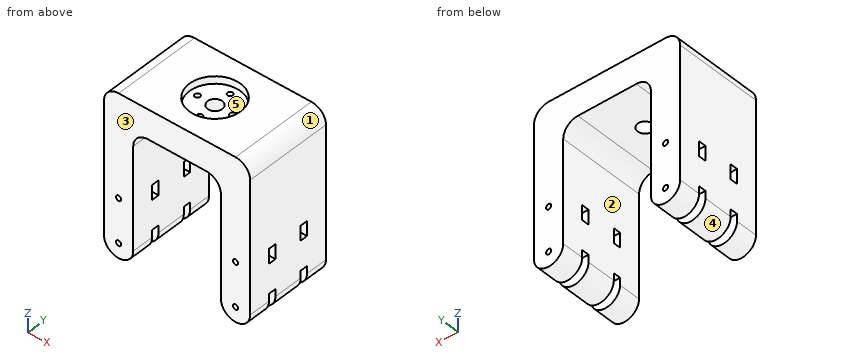
```python
from build123d import *

# Parameters (mm, degrees)
BOSS_EXTRUDE1_DEPTH     = 30
FILLET1_R               = 10
CUT_EXTRUDE1_DEPTH      = 125.49899598
CUT_EXTRUDE1_DEPTH_BACK = 125.49899598
SKETCH3_R               = 5
SKETCH4_R               = 17.5
CUT_EXTRUDE2_DEPTH      = 5
SKETCH5_R               = 1.8
CUT_EXTRUDE3_DEPTH      = 5
CIRPATTERN1_COUNT       = 4
SKETCH6_R               = 1.8
CUT_EXTRUDE4_DEPTH      = 135.907375632
SKETCH7_W               = 20
SKETCH7_H               = 10
CUT_EXTRUDE5_DEPTH      = 5
MIRROR2_COPY_1_SKETCH_W = 20
MIRROR2_COPY_1_SKETCH_H = 10
MIRROR2_COPY_1_DEPTH    = 5


with BuildPart() as part:
    # Sketch1 → Boss-Extrude1 (new, symmetric)
    with BuildSketch(Plane(origin=(0, 0, 0), x_dir=(1, 0, 0), z_dir=(0, 1, 0))):
        with BuildLine():
            Line((-50, 0), (50, 0))
            Line((50, 0), (50, 100))
            ThreePointArc((50, 100), (40, 110), (30, 100))
            Line((30, 100), (30, 20))
            Line((30, 20), (-30, 20))
            Line((-30, 20), (-30, 100))
            ThreePointArc((-30, 100), (-40, 110), (-50, 100))
            Line((-50, 100), (-50, 0))
        make_face()
    extrude(amount=BOSS_EXTRUDE1_DEPTH, both=True)

    # Fillet1
    fillet1_edges = [part.edges().sort_by_distance(p)[0] for p in [
        (50, 0, 0),
        (-50, 0, 0),
        (-30, 0, -20),
        (30, 0, -20),
    ]]
    fillet(fillet1_edges, radius=FILLET1_R)

    # Sketch3 → Cut-Extrude1 (cut, two sides: drawn at the far end of the back side and taken through both)
    with BuildSketch(Plane.XY.offset(-CUT_EXTRUDE1_DEPTH_BACK)):
        Circle(SKETCH3_R)
    extrude(amount=CUT_EXTRUDE1_DEPTH + CUT_EXTRUDE1_DEPTH_BACK, mode=Mode.SUBTRACT)

    # Sketch4 → Cut-Extrude2 (cut)
    with BuildSketch(Plane.XY):
        Circle(SKETCH4_R)
    extrude(amount=-CUT_EXTRUDE2_DEPTH, mode=Mode.SUBTRACT)

    # Sketch5 → Cut-Extrude3 (cut)
    with BuildSketch(Plane.XY.offset(-5)):
        with Locations((0, -12)):
            Circle(SKETCH5_R)
    cut_extrude3 = extrude(amount=-CUT_EXTRUDE3_DEPTH, mode=Mode.SUBTRACT)

    # CirPattern1: Cut-Extrude3 ×4 about axis
    cirpattern1_axis = Axis((0, 0, 0), (0, 0, 1))
    for i in range(1, CIRPATTERN1_COUNT):
        add(cut_extrude3.rotate(cirpattern1_axis, i * 360 / CIRPATTERN1_COUNT), mode=Mode.SUBTRACT)

    # Sketch6 → Cut-Extrude4 (cut, through all)
    with BuildSketch(Plane(origin=(0, 30, 0), x_dir=(1, 0, 0), z_dir=(0, 1, 0))):
        with Locations(Location((-40, 100, 0), (0, 0, 270))):
            Circle(SKETCH6_R)
        with Locations(Location((-40, 70, 0), (0, 0, 270))):
            Circle(SKETCH6_R)
    cut_extrude4 = extrude(amount=-CUT_EXTRUDE4_DEPTH, mode=Mode.SUBTRACT)

    # Sketch7 → Cut-Extrude5 (cut)
    with BuildSketch(Plane(origin=(0, 15, 0), x_dir=(1, 0, 0), z_dir=(0, 1, 0))):
        with BuildLine():
            Line((-50, 105), (-50, 95))
            Line((-50, 95), (-30, 95))
            Line((-30, 95), (-30, 105))
            ThreePointArc((-30, 105), (-40, 115), (-50, 105))
        make_face()
        with Locations((-40, 70)):
            Rectangle(SKETCH7_W, SKETCH7_H)
    cut_extrude5 = extrude(amount=-CUT_EXTRUDE5_DEPTH, mode=Mode.SUBTRACT)

    # Mirror1: Cut-Extrude5 across plane
    add(cut_extrude5.mirror(Plane.ZX), mode=Mode.SUBTRACT)

    # Mirror2: Cut-Extrude4, Cut-Extrude5 across plane
    add(cut_extrude4.mirror(Plane(origin=(0, 0, 0), x_dir=(0, 0, 1), z_dir=(1, 0, 0))), mode=Mode.SUBTRACT)
    add(cut_extrude5.mirror(Plane(origin=(0, 0, 0), x_dir=(0, 0, 1), z_dir=(1, 0, 0))), mode=Mode.SUBTRACT)

    # Mirror2 copy 1 sketch → Mirror2 copy 1 (cut)
    with BuildSketch(Plane(origin=(0, -15, 0), x_dir=(-1, 0, 0), z_dir=(0, -1, 0))):
        with BuildLine():
            Line((-50, 105), (-50, 95))
            Line((-50, 95), (-30, 95))
            Line((-30, 95), (-30, 105))
            ThreePointArc((-30, 105), (-40, 115), (-50, 105))
        make_face()
        with Locations((-40, 70)):
            Rectangle(MIRROR2_COPY_1_SKETCH_W, MIRROR2_COPY_1_SKETCH_H)
    extrude(amount=-MIRROR2_COPY_1_DEPTH, mode=Mode.SUBTRACT)


solid = part.part
```
Work out the finished part from the listing and answer in its coordinate system (mm). Face numbers are marked on the shaded views. A direction names the side the tool comes from. Round coordinates to 2 decimals unless told otherwise and drop trailing zeros. Order: outer loops, then holes, each group sorted by start corner. A loop starts at its lowest first (then second) coordinate and runs counter-clockwise, first axis right, second up.
Q1. A tool of negligible diameter and unlimited length cuts with its end or side. For the marked faces 1 and 2, from which of +Z, -Z, +X, -X, +Y, -Y can it reach the whole face along a straight path? Write none if from no direction.
Solution:
face 1: +Z, +X, +Y, -Y
face 2: -Z, +Y, -Y
Q2. The mould has two halves that part along Y. Classify the marked faces 3, 4 and 5: pulls with the +Y half, pulls with the -Y half, needs draft (parallel to the pull), parting line crosses it, or undercut.
Solution:
face 3: pulls with the -Y half
face 4: needs draft
face 5: undercut
Q3. Given pin 1 Ø1.8 at (x, y) = (0.5, 11.5) entering from +Z; pin 2 Ø3 at (x, z) = (-40, -100) entering from -Y; pin 3 Ø1.5 at (x, y) = (-42, 12.5) entering from -Z; pin 4 Ø4 at (x, y) = (-44, 11.5) entering from -Z (3 decimals), each flat-ended and moving along its own axis, determine where each tip first touches the part or whether it passes through.
Solution:
pin 1: stops at z = -10
pin 2: passes through
pin 3: stops at z = -95
pin 4: stops at z = -109.635
Q4. A cutting plane is placed at C-C, the plane z = -53.5. Determine the outline of the cut face in (x, y).
Solution:
outline: (-50, -30) - (-30, -30) - (-30, 30) - (-50, 30) - close; (30, -30) - (50, -30) - (50, 30) - (30, 30) - close
Q5. Find the intervals of material crossed by line 1 along X through (y, z) = (24.75, -70); line 2 along Y through (x, z) = (0, -7); line 3 along Y through (x, z) = (30.5, -100), in increasing order.
Solution:
line 1: x = -50 to -41.8, -38.2 to -30, 30 to 38.2, 41.8 to 50
line 2: y = -30 to -13.8, -10.2 to -5, 5 to 10.2, 13.8 to 30
line 3: y = -30 to -15, -10 to 10, 15 to 30
Q6. A cutting plane is placed at B-B, the plane x = 0. Determine the outline of the cut face in (y, z), then the cut area to 3 significant figures.
Solution:
outline: (-30, -20) - (-5, -20) - (-5, -5) - (-10.2, -5) - (-10.2, -10) - (-13.8, -10) - (-13.8, -5) - (-17.5, -5) - (-17.5, 0) - (-30, 0) - close; (5, -20) - (30, -20) - (30, 0) - (17.5, 0) - (17.5, -5) - (13.8, -5) - (13.8, -10) - (10.2, -10) - (10.2, -5) - (5, -5) - close
area: 839 mm2
Q7. A cutting plane is placed at A-A, the plane y = 0. Count the separate pieces of the cut face and the enclosed holes in it, then the cut area to 3 significant figures.
Solution:
separate pieces: 2
enclosed holes: 4
area: 5,110 mm2
Q8. A cutting plane is placed at D-D, the plane y = 23.5. Determine the outline of the cut face in (x, z).
Solution:
outline: (-50, -100) arc R10 ccw to (-30, -100) - (-30, -30) arc R10 cw to (-20, -20) - (20, -20) arc R10 cw to (30, -30) - (30, -100) arc R10 ccw to (50, -100) - (50, -10) arc R10 ccw to (40, 0) - (-40, 0) arc R10 ccw to (-50, -10) - close; hole circle Ø3.6 at (-40, -100); hole circle Ø3.6 at (-40, -70); hole circle Ø3.6 at (40, -100); hole circle Ø3.6 at (40, -70)
